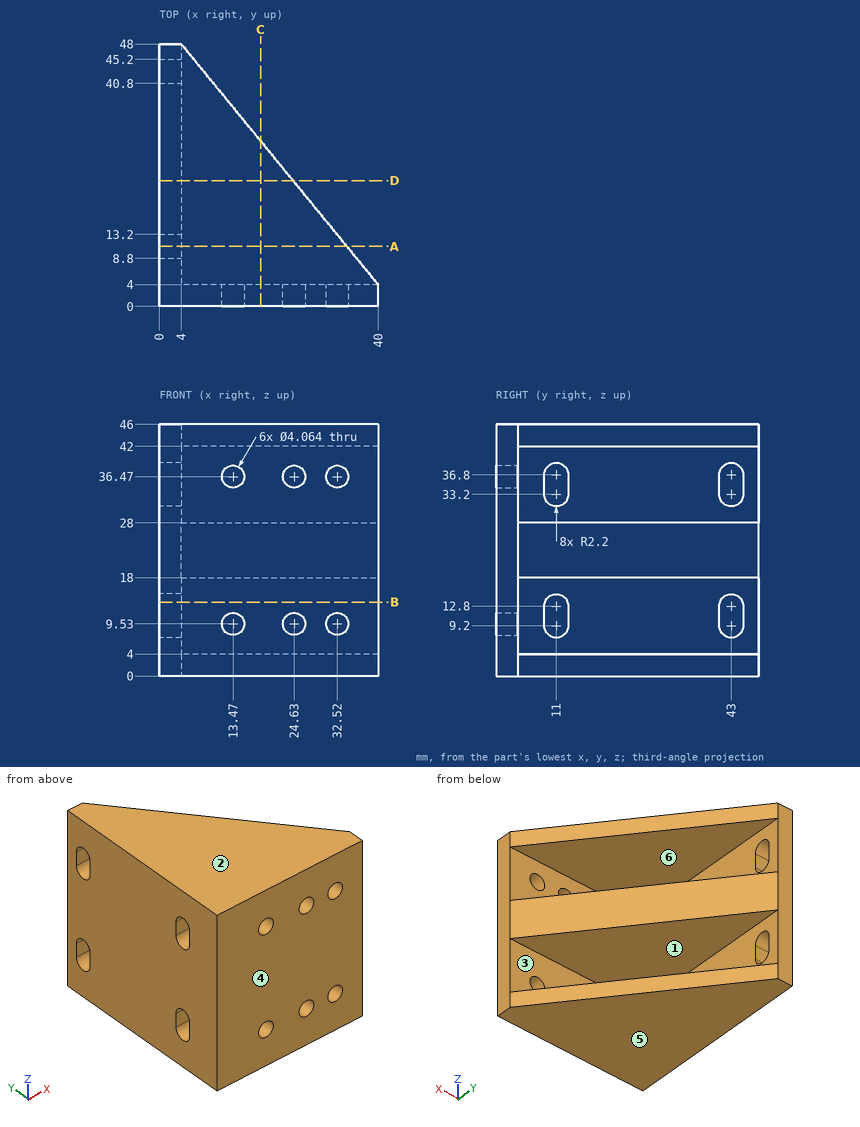
The figure shows three views and two pictorial views of one solid part (mm, origin at its lowest corner). Answer the questions. A direction names the side the tool comes from. Coordinates: 2 decimals unless noted, no trailing zeros. Write each loop counter-clockwise with the first axis right and the second up, starting at its lowest first coordinate (ties: lowest second). Pieces come first, ordered by that corner, then holes. Notation, with made-up numbers: (21, -10) -> (53, -10) arc R23 cw to (53, 18) -> close; hole circle Ø7 at (20, 0.25). An arc over 180 degrees is marked (long way). Return JSON: item names as keys, results as strings.
(1) The part is cut by section C-C on x = 18.5. Give the vertices of the cut face in (y, z), then the cut area to 3 significant figures.
Answers below:
{"outline": "(0, 0) -> (30.28, 0) -> (30.28, 4) -> (4, 4) -> (4, 18) -> (30.28, 18) -> (30.28, 28) -> (4, 28) -> (4, 42) -> (30.28, 42) -> (30.28, 46) -> (0, 46) -> close", "area": "657 mm^2"}
(2) For a pull along Z with two mould halves and no side action, classify the marked faces 3, 4, 5 and 6 as pulls with the +Z half, pulls with the -Z half, needs draft (parallel to the pull), parting line crosses it, or undercut.
Answers below:
{"face 3": "undercut", "face 4": "needs draft", "face 5": "pulls with the -Z half", "face 6": "undercut"}
(3) The part is cut by section A-A on y = 11. Give the vertices of the cut face in (x, z).
Answers below:
{"outline": "(0, 0) -> (34.27, 0) -> (34.27, 4) -> (4, 4) -> (4, 7) -> (0, 7) -> close; (0, 15) -> (4, 15) -> (4, 18) -> (34.27, 18) -> (34.27, 28) -> (4, 28) -> (4, 31) -> (0, 31) -> close; (0, 39) -> (4, 39) -> (4, 42) -> (34.27, 42) -> (34.27, 46) -> (0, 46) -> close"}
(4) The part is cut by section D-D on y = 23. Give the vertices of the cut face in (x, z) (1 decimal).
Answers below:
{"outline": "(0, 0) -> (24.5, 0) -> (24.5, 4) -> (4, 4) -> (4, 18) -> (24.5, 18) -> (24.5, 28) -> (4, 28) -> (4, 42) -> (24.5, 42) -> (24.5, 46) -> (0, 46) -> close"}
(5) Which of the six approach directions +Z, -Z, +X, -X, +Y, -Y give full straight-line access (tool end or side, diameter ignored) to the marked faces 1 and 2?
Answers below:
{"face 1": "+X, +Y", "face 2": "+Z, +X, -X, +Y, -Y"}
(6) The part is cut by section B-B on z = 13.5. Give the vertices of the cut face in (x, y) (1 decimal).
Answers below:
{"outline": "(0, 0) -> (40, 0) -> (40, 4) -> (4, 4) -> (4, 8.9) -> (0, 8.9) -> close; (0, 13.1) -> (4, 13.1) -> (4, 40.9) -> (0, 40.9) -> close; (0, 45.1) -> (4, 45.1) -> (4, 48) -> (0, 48) -> close"}
(7) Consider line 1 along Z through (x, y) = (4.5, 39); line 2 along Y through (x, z) = (18, 29). Determine where each line is inside the solid, lowest interval first. Write a range as from..to.
Answers below:
{"line 1": "0..4, 18..28, 42..46", "line 2": "0..4"}
(8) Each of these flat-tipped pins is pushed along its axis until it touches: P1, Ø7, axis at y = 26, z = 38, coming from the +X side; P2, Ø8, axis at y = 28, z = 17.5, coming from the +X side; P3, Ø4, axis at x = 21.5, z = 37.5, coming from the +Y side. Where does it stop, or does it pass through?
Answers below:
{"P1": "x = 4", "P2": "x = 23.61", "P3": "y = 4"}
